from build123d import *

# Parameters (mm, degrees)
F1_DEPTH = 1000


with BuildPart() as f1:
    # F0 (on Front) → F1 (new body)
    with BuildSketch(Plane.XZ):
        with BuildLine():
            Line((-33.991796, -5.594154), (-33.991796, -10.594154))
            Line((-33.991796, -10.594154), (6.008204, -10.594154))
            Line((6.008204, -10.594154), (6.008204, -5.594154))
            Line((6.008204, -5.594154), (-4.741796, -5.594154))
            Line((-4.741796, -5.594154), (-4.741796, 1.051143))
            Line((-4.741796, 1.051143), (-9.991796, 1.051143))
            Line((-9.991796, 1.051143), (-9.991796, 7.205846))
            Line((-9.991796, 7.205846), (-10.504677, 7.205846))
            ThreePointArc((-10.504677, 7.205846), (-13.991796, 22.405846), (-17.478915, 7.205846))
            Line((-17.478915, 7.205846), (-17.991796, 7.205846))
            Line((-17.991796, 7.205846), (-17.991796, 1.051143))
            Line((-17.991796, 1.051143), (-23.241796, 1.051143))
            Line((-23.241796, 1.051143), (-23.241796, -5.594154))
            Line((-23.241796, -5.594154), (-33.991796, -5.594154))
        make_face()
    extrude(amount=F1_DEPTH)


solid = f1.part
Read the model definition and answer for the solid it produces. Units are mm, in the model's axes. Coordinates: 2 decimals unless noted, no trailing zeros. Loops run counter-clockwise (first coordinate to the right, second up) from the corner with the lowest first, then second, coordinate; pieces in that order, holes last.
Q1. The part is cut by section A-A on y = -227. Write down the section's boundary in (x, z).
Q2. The part is cut by section B-B on z = 17. Write down the section's boundary in (x, y).
Q3. The mould has two halves that part along Z. Classify faces 1 (the face through (-14, -493, -10.594)), 2 (the face through (-14, -1000, 2)), 3 (the face through (-13.7, -493, 22.4)): +Z half, -Z half, draft (parallel to the pull), parting line (faces both ways), or undercut.
Q4. Consider probe 1 along Z at (x, y) = (-25, -906.5); probe 2 along X at (y, z) = (-631, 1); probe 3 along X at (y, z) = (-268, 13). Determine where each line is inside the solid, lowest interval first.
Q5. Each of these flat-tipped pins is pushed along its axis until it touches: pin 1 Ø3.5 at (y, z) = (-445.5, -2) entering from +X; pin 2 Ø1.5 at (y, z) = (-451.5, 6) entering from -X; pin 3 Ø0.6 at (x, y) = (-10, -317) entering from +Z; pin 4 Ø5.5 at (y, z) = (-311, -3.5) entering from -X. Where does it stop, or does it pass through?
Results below:
1. outline: (-33.99, -10.59) - (6.01, -10.59) - (6.01, -5.59) - (-4.74, -5.59) - (-4.74, 1.05) - (-9.99, 1.05) - (-9.99, 7.21) - (-10.5, 7.21) arc R8 ccw (long way) to (-17.48, 7.21) - (-17.99, 7.21) - (-17.99, 1.05) - (-23.24, 1.05) - (-23.24, -5.59) - (-33.99, -5.59) - close
2. outline: (-21.56, -1000) - (-6.42, -1000) - (-6.42, 0) - (-21.56, 0) - close
3. face 1: -Z half
3. face 2: draft
3. face 3: undercut
4. probe 1: z = -10.59 to -5.59
4. probe 2: x = -23.24 to -4.74
4. probe 3: x = -21.87 to -6.12
5. pin 1: stops at x = -4.74
5. pin 2: stops at x = -17.99
5. pin 3: stops at z = 21.5
5. pin 4: stops at x = -33.99
